```python
from build123d import *

# Parameters (mm, degrees)
SKETCH1_W             = 10
SKETCH1_H             = 32
BOSS_EXTRUDE1_DEPTH   = 30
M4_TAPPED_HOLE1_D     = 3.3
M4_TAPPED_HOLE1_DEPTH = 10.1
M4_TAPPED_HOLE1_TIP   = 0.991420021
SKETCH4_R             = 5.5
CUT_EXTRUDE2_DEPTH    = 10


with BuildPart() as part:
    # Sketch1 → Boss-Extrude1 (new body)
    with BuildSketch(Plane(origin=(0, 0, 0), x_dir=(0, 0, -1), z_dir=(1, 0, 0))):
        with Locations((5, 16)):
            Rectangle(SKETCH1_W, SKETCH1_H)
    extrude(amount=BOSS_EXTRUDE1_DEPTH)

    # M4 Tapped Hole1
    with Locations(Plane(origin=(0, 0, 0), x_dir=(-1, 0, 0), z_dir=(0, -1, 0))):
        with Locations((-5, 5), (-25, 5)):
            Hole(M4_TAPPED_HOLE1_D / 2, depth=M4_TAPPED_HOLE1_DEPTH)
            with Locations((0, 0, -(M4_TAPPED_HOLE1_DEPTH + M4_TAPPED_HOLE1_TIP / 2))):  # 118° drill point
                Cone(0, M4_TAPPED_HOLE1_D / 2, M4_TAPPED_HOLE1_TIP, mode=Mode.SUBTRACT)

    # Sketch4 → Cut-Extrude2 (cut)
    with BuildSketch(Plane.XY):
        with Locations((15, 17)):
            Circle(SKETCH4_R)
    extrude(amount=-CUT_EXTRUDE2_DEPTH, mode=Mode.SUBTRACT)


solid = part.part
```
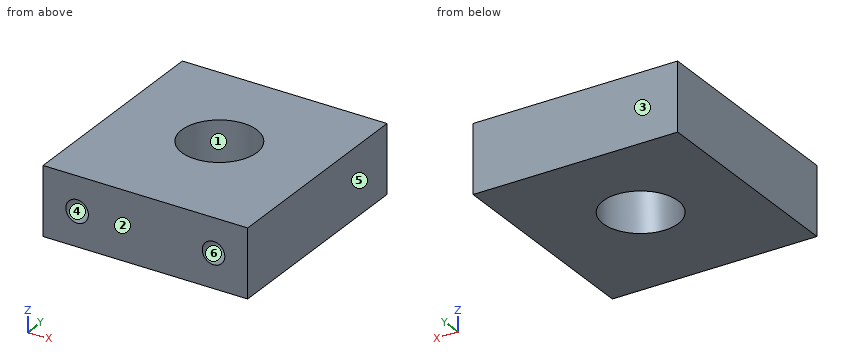
Here's how the part is built. I have some questions about the finished solid (model axes, mm). Face numbers are marked on the shaded views. A direction names the side the tool comes from. Give positions to 0.01 mm unless a question says otherwise; leave off trailing zeros. Loops run counter-clockwise (first coordinate to the right, second up) from the corner with the lowest first, then second, coordinate; pieces in that order, holes last. Notation, with made-up numbers: M 8.25,69 L 21.25,69 A17 ccw 21.25,96 Z; hole C 18.5,-23.5 d4. An arc over 180 degrees is marked long. Use one line per item in the form item = value. Start each with the question number.
Q1. I need wall thicknesses on line 1 along X through (y, z) = (7.75, -5); line 2 along Z through (x, y) = (25, 4); line 3 along Y through (x, z) = (15, -2.5). Which ranges of each line are inside material? Lowest first, please.
Q2. If we section it at B-B (z = -7.25): Write out the boundary of the cut face in (x, y), then the cut area to 3 significant figures.
Q3. Which directions (+Z, -Z, +X, -X, +Y, -Y) give clear straight access to the entire face, cutting with the end or side of a thin tool? Please do the marked faces 5 and 6.
Q4. If we section it at C-C (y = 17): Write out the boundary of the cut face in (x, z).
Q5. Thinking about a two-plate mould opening in Y: for the marked faces 1, 2, 3 and 4, which applies, +Y half, -Y half, draft (parallel to the pull), parting line (faces both ways), or undercut?
Q6. If we section it at D-D (y = 3.5): Write out the boundary of the cut face in (x, z).
Q7. If we section it at A-A (x = 15): Write out the boundary of the cut face in (y, z).
Taken from the geometry:
q1.line_1 = 0 to 3.35, 6.65 to 23.35, 26.65 to 30
q1.line_2 = -10 to -6.65, -3.35 to 0
q1.line_3 = 0 to 11.5, 22.5 to 32
q2.outline = M 0,0 L 30,0 L 30,32 L 0,32 Z; hole C 15,17 d11
q2.area = 865 mm^2
q3.face_5 = +Z, -Z, +X, +Y, -Y
q3.face_6 = -Y
q4.outline = M 0,-10 L 9.5,-10 L 9.5,0 L 0,0 Z; M 20.5,-10 L 30,-10 L 30,0 L 20.5,0 Z
q5.face_1 = undercut
q5.face_2 = -Y half
q5.face_3 = +Y half
q5.face_4 = draft
q6.outline = M 0,-10 L 30,-10 L 30,0 L 0,0 Z; hole C 5,-5 d3.3; hole C 25,-5 d3.3
q7.outline = M 0,-10 L 11.5,-10 L 11.5,0 L 0,0 Z; M 22.5,-10 L 32,-10 L 32,0 L 22.5,0 Z
